Source: CAD feature listing. Evaluate the final solid. Frame: model axes, mm. A direction names the side the tool comes from. Round coordinates to 2 decimals unless told otherwise and drop trailing zeros. Loops run counter-clockwise (first coordinate to the right, second up) from the corner with the lowest first, then second, coordinate; pieces in that order, holes last. Notation, with made-up numbers: M -7.5,14.5 L 44.5,14.5 A23 ccw 44.5,38.5 Z; hole C -28.5,89 d11. An arc over 180 degrees is marked long. Write each question's results on one line, items separated by ' | '. Start each with the question number.
1. Ray query, line 1 (X direction, y = -8.3, z = 0); line 2 (X direction, y = -7, z = -0.75); line 3 (X direction, y = 7.2, z = 0). Return the intervals inside material, ascending.
2. Section A-A on y = -7. Output: boundary loops of the cut face in (x, z), and give its area (3 significant figures).
3. Section B-B on x = -17. Output: boundary loops of the cut face in (y, z), and give its area (3 significant figures).
4. Section C-C on x = 14. Output: boundary loops of the cut face in (y, z).
5. Draft query along Z for faces 1 (the flat face through (-18, -6, 3)), 2 (the flat face through (3, -3, 7.5)), 3 (the flat face through (12, 8, 2)). Return one class per face: released by +Z, released by -Z, zero draft, split by the parting line, or undercut.
6. Contact query for flat-ended pins moving along their axis: pin 1 Ø1 at (x, z) = (-13, -2) entering from +Y; pin 2 Ø2.5 at (x, z) = (10, 0) entering from +Y; pin 3 Ø8 at (y, z) = (2, 4) entering from -X; pin 4 Ø6 at (y, z) = (5.5, 2.5) entering from -X. Output: stop coordinate, or through.
7. Set-up query: faces 4 (the cylindrical face through (-11.05, -8.54, 0.78)), 5 (the cylindrical face through (12.32, 1.95, -6.2)), 6 (the flat face through (-21, -2.5, 0)). Return all of +Z, -Z, +X, -X, +Y, -Y with unobstructed straight access to the full face (end or side cutting, diameter ignored); none if empty.
from build123d import *

# Parameters (mm, degrees)
SKETCH1_W               = 15
SKETCH1_H               = 19
SKETCH1_R               = 6.5
BOSS_EXTRUDE1_DEPTH     = 25
SKETCH2_W               = 15
SKETCH2_H               = 19
BOSS_EXTRUDE2_DEPTH     = 2
CUT_EXTRUDE1_DEPTH      = 29.324018077
CUT_EXTRUDE1_DEPTH_BACK = 29.324018077
SKETCH4_R               = 2
SKETCH3_W               = 28
SKETCH3_H               = 15
SKETCH3_R               = 3
BOSS_EXTRUDE3_DEPTH     = 8.5
CHAMFER1_SIZE2          = 10.5
CHAMFER1_SIZE           = 4
SKETCH7_R               = 6
CUT_EXTRUDE4_DEPTH      = 5


with BuildPart() as part:
    # Sketch1 → Boss-Extrude1 (new body)
    with BuildSketch(Plane(origin=(0, 0, 0), x_dir=(0, 0, -1), z_dir=(1, 0, 0))):
        with Locations((0, -1.5)):
            Rectangle(SKETCH1_W, SKETCH1_H)
        Circle(SKETCH1_R, mode=Mode.SUBTRACT)
    extrude(amount=BOSS_EXTRUDE1_DEPTH)

    # Sketch2 → Boss-Extrude2 (add)
    with BuildSketch(Plane(origin=(0, 0, 0), x_dir=(0, 0, -1), z_dir=(1, 0, 0))):
        with Locations((0, -1.5)):
            Rectangle(SKETCH2_W, SKETCH2_H)
    extrude(amount=-BOSS_EXTRUDE2_DEPTH)

    # Sketch4 → Cut-Extrude1 (cut, two sides: drawn at the far end of the back side and taken through both)
    with BuildSketch(Plane(origin=(0, 0, 0), x_dir=(1, 0, 0), z_dir=(0, 1, 0)).offset(-CUT_EXTRUDE1_DEPTH_BACK)):
        with Locations(Location((10, 0, 0), (0, 0, 270))):
            Circle(SKETCH4_R)
        with Locations(Location((20, 0, 0), (0, 0, 270))):
            Circle(SKETCH4_R)
    extrude(amount=CUT_EXTRUDE1_DEPTH + CUT_EXTRUDE1_DEPTH_BACK, mode=Mode.SUBTRACT)

    # Sketch3 → Boss-Extrude3 (add)
    with BuildSketch(Plane(origin=(0, -2.5, 0), x_dir=(1, 0, 0), z_dir=(0, 1, 0))):
        with Locations((-16, 0)):
            Rectangle(SKETCH3_W, SKETCH3_H)
        with Locations(Location((-17, 0, 0), (0, 0, 270))):
            Circle(SKETCH3_R, mode=Mode.SUBTRACT)
    extrude(amount=-BOSS_EXTRUDE3_DEPTH)

    # Chamfer1
    chamfer1_edges = [part.edges().sort_by_distance(p)[0] for p in [
        (-2, -2.5, 0),
    ]]
    chamfer1_side = [part.faces().sort_by_distance(p)[0] for p in [
        (-2.08, -2.5, 0),
    ]]
    chamfer(chamfer1_edges, length=CHAMFER1_SIZE - 0.0001, length2=CHAMFER1_SIZE2 - 0.0001, reference=chamfer1_side[0])  # a hair under: the kernel refuses the full size

    # Sketch7 → Cut-Extrude4 (cut)
    with BuildSketch(Plane.XZ.offset(11)):
        with Locations(Location((-17, 0, 0), (0, 0, 270))):
            Circle(SKETCH7_R)
    extrude(amount=-CUT_EXTRUDE4_DEPTH, mode=Mode.SUBTRACT)


solid = part.part
Taken from the geometry:
1) line 1: -30 to -23, -11 to 8, 12 to 18, 22 to 25 | line 2: -30 to -22.95, -11.05 to 8.15, 11.85 to 18.15, 21.85 to 25 | line 3: -2.3 to 8, 12 to 18, 22 to 25
2) outline: M -30,-7.5 L 25,-7.5 L 25,7.5 L -30,7.5 Z; hole C -17,0 d12; hole C 10,0 d4; hole C 20,0 d4 | area: 687 mm^2
3) outline: M -11,-7.5 L -2.5,-7.5 L -2.5,-3 L -6,-3 L -6,-6 L -11,-6 Z; M -11,6 L -6,6 L -6,3 L -2.5,3 L -2.5,7.5 L -11,7.5 Z | area: 46.5 mm^2
4) outline: M -11,-7.5 L 8,-7.5 L 8,7.5 L -11,7.5 Z; hole C 0,0 d13
5) face 1: undercut | face 2: released by +Z | face 3: zero draft
6) pin 1: y = -2.5 | pin 2: through | pin 3: x = -5.81 | pin 4: x = -4.1
7) face 4: -Y | face 5: +X | face 6: +Z, -Z, -X, +Y
